```python
from build123d import *

# Parameters (mm, degrees)
SKETCH1_W            = 87.8
SKETCH1_H            = 71.8
BOSS_EXTRUDE1_DEPTH  = 2.6
CUT_EXTRUDE1_DEPTH   = 3.6
SKETCH4_R            = 3.3
CUT_EXTRUDE2_DEPTH   = 3.6
SKETCH3_R            = 2.4
BOSS_EXTRUDE2_DEPTH  = 1.6
LPATTERN1_COUNT      = 9
LPATTERN1_PITCH      = 8
LPATTERN1_COUNT_DIR2 = 11
LPATTERN1_PITCH_DIR2 = 8


with BuildPart() as part:
    # Sketch1 → Boss-Extrude1 (new body)
    with BuildSketch(Plane.XY):
        Rectangle(SKETCH1_W, SKETCH1_H)
    extrude(amount=BOSS_EXTRUDE1_DEPTH)

    # Sketch2 → Cut-Extrude1 (cut, through all)
    with BuildSketch(Plane.XY):
        with BuildLine():
            Line((-8, 12), (8, 12))
            ThreePointArc((8, 12), (10.828427125, 10.828427125), (12, 8))
            Line((12, 8), (12, -8))
            ThreePointArc((12, -8), (10.828427125, -10.828427125), (8, -12))
            Line((8, -12), (-8, -12))
            ThreePointArc((-8, -12), (-10.828427125, -10.828427125), (-12, -8))
            Line((-12, -8), (-12, 8))
            ThreePointArc((-12, 8), (-10.828427125, 10.828427125), (-8, 12))
        make_face()
    extrude(amount=CUT_EXTRUDE1_DEPTH, mode=Mode.SUBTRACT)

    # Sketch4 → Cut-Extrude2 (cut, through all)
    with BuildSketch(Plane.XY.offset(2.6)):
        with Locations((-23.75, -17.7)):
            Circle(SKETCH4_R)
    cut_extrude2 = extrude(amount=-CUT_EXTRUDE2_DEPTH, mode=Mode.SUBTRACT)

    # Mirror1: Cut-Extrude2 across plane
    add(cut_extrude2.mirror(Plane(origin=(0, 0, 0), x_dir=(0, 0, 1), z_dir=(1, 0, 0))), mode=Mode.SUBTRACT)

    # Sketch3 → Boss-Extrude2 (add)
    with BuildSketch(Plane.XY.offset(2.6)):
        with Locations((-40, -32)):
            Circle(SKETCH3_R)
    boss_extrude2 = extrude(amount=BOSS_EXTRUDE2_DEPTH)

    # LPattern1: Boss-Extrude2 9 × 11, 23 skipped
    with Locations(*[(j * LPATTERN1_PITCH_DIR2, i * LPATTERN1_PITCH, 0) for i in range(LPATTERN1_COUNT) for j in range(LPATTERN1_COUNT_DIR2) if (i, j) not in ((0, 0), (2, 2), (2, 4), (2, 5), (2, 6), (2, 8), (3, 3), (3, 4), (3, 5), (3, 6), (3, 7), (4, 3), (4, 4), (4, 5), (4, 6), (4, 7), (5, 3), (5, 4), (5, 5), (5, 6), (5, 7), (6, 4), (6, 5), (6, 6))]):
        add(boss_extrude2)


solid = part.part
```
Read the model definition and answer for the solid it produces. Units are mm, in the model's axes. A direction names the side the tool comes from. Coordinates: 2 decimals unless noted, no trailing zeros. Loops run counter-clockwise (first coordinate to the right, second up) from the corner with the lowest first, then second, coordinate; pieces in that order, holes last.
(1) The part is cut by section B-B (z = 1.5). Determine the outline of the cut face in (x, y), and give its area (3 significant figures).
Solution:
outline: (-43.9, -35.9) - (43.9, -35.9) - (43.9, 35.9) - (-43.9, 35.9) - close; hole circle Ø6.6 at (-23.75, -17.7); hole (-12, -8) arc R4 ccw to (-8, -12) - (8, -12) arc R4 ccw to (12, -8) - (12, 8) arc R4 ccw to (8, 12) - (-8, 12) arc R4 ccw to (-12, 8) - close; hole circle Ø6.6 at (23.75, -17.7)
area: 5,670 mm2
(2) The part is cut by section D-D (x = 36.5). Determine the outline of the cut face in (y, z), and give its area (3 significant figures).
Solution:
outline: (-35.9, 0) - (35.9, 0) - (35.9, 2.6) - (-35.9, 2.6) - close
area: 187 mm2
(3) The mould has two halves that part along X. Classify faces 3 (the face through (-1, -35.9, 1)), 4 (the face through (20.7, -18.96, 1.32)), 5 (the face through (21.602, 8.106, 3.389)): released by +X, released by -X, zero draft, split by the parting line, or undercut.
Solution:
face 3: zero draft
face 4: undercut
face 5: undercut
(4) A tool of negligible diameter and unlimited length cuts with its end or side. For faces 1 (the face through (-34.398, -15.894, 3.389)), 2 (the face through (40, 16, 4.2)), from which of +Z, -Z, +X, -X, +Y, -Y can it reach the whole face along a straight path? Write none if from no direction.
Solution:
face 1: +Z
face 2: +Z, +X, -X, +Y, -Y
(5) A flat-ended cylindrical pin translates along its axis: pin 1 Ø2 at (x, y) = (-33.5, -20.5) entering from +Z. Find the tip coordinate at first contact, or state that the pin passes through.
Solution:
pin 1: stops at z = 2.6
(6) The part is cut by section A-A (x = 0). Determine the outline of the cut face in (y, z), and give its area (3 significant figures).
Solution:
outline: (-35.9, 0) - (-12, 0) - (-12, 2.6) - (-21.6, 2.6) - (-21.6, 4.2) - (-26.4, 4.2) - (-26.4, 2.6) - (-29.6, 2.6) - (-29.6, 4.2) - (-34.4, 4.2) - (-34.4, 2.6) - (-35.9, 2.6) - close; (12, 0) - (35.9, 0) - (35.9, 2.6) - (34.4, 2.6) - (34.4, 4.2) - (29.6, 4.2) - (29.6, 2.6) - (26.4, 2.6) - (26.4, 4.2) - (21.6, 4.2) - (21.6, 2.6) - (12, 2.6) - close
area: 155 mm2
(7) The part is cut by section C-C (x = -16.5). Determine the outline of the cut face in (y, z).
Solution:
outline: (-35.9, 0) - (35.9, 0) - (35.9, 2.6) - (34.35, 2.6) - (34.35, 4.2) - (29.65, 4.2) - (29.65, 2.6) - (26.35, 2.6) - (26.35, 4.2) - (21.65, 4.2) - (21.65, 2.6) - (18.35, 2.6) - (18.35, 4.2) - (13.65, 4.2) - (13.65, 2.6) - (-13.65, 2.6) - (-13.65, 4.2) - (-18.35, 4.2) - (-18.35, 2.6) - (-21.65, 2.6) - (-21.65, 4.2) - (-26.35, 4.2) - (-26.35, 2.6) - (-29.65, 2.6) - (-29.65, 4.2) - (-34.35, 4.2) - (-34.35, 2.6) - (-35.9, 2.6) - close
(8) Consider line 1 along Y through (x, z) = (16, 2.7); line 2 along Y through (x, z) = (-23.75, 0.65); line 3 along X through (y, z) = (-4.5, 1.2). Determine where each line is inside the solid, lowest interval first.
Solution:
line 1: y = -34.4 to -29.6, -26.4 to -21.6, -18.4 to -13.6, 13.6 to 18.4, 21.6 to 26.4, 29.6 to 34.4
line 2: y = -35.9 to -21, -14.4 to 35.9
line 3: x = -43.9 to -12, 12 to 43.9
